Build history of the part. All positions in model axes, mm. A direction names the side the tool comes from. Give positions to 0.01 mm unless a question says otherwise; leave off trailing zeros. Order: outer loops, then holes, each group sorted by start corner. A loop starts at its lowest first (then second) coordinate and runs counter-clockwise, first axis right, second up. Notation, with made-up numbers: (34.5, -29.75) - (78.5, -29.75) arc R11 ccw to (78.5, -23.75) - close; hole circle Ø2 at (26, 79.5). An arc over 180 degrees is marked (long way). Use a Markdown table: item, result. Add a question column.
(1) Flat gauge pins, fed straight in: pin 1 (2 mm diameter, centred on y = 2.5, z = 2.5, fed in from -X); pin 2 (2 mm diameter, centred on y = -2, z = 3, fed in from -X); pin 3 (1.5 mm diameter, centred on y = 12.5, z = 2.5, fed in from -X). Where does each tip first touch, or does it go through?
(2) Which spindle directions (+Z, -Z, +X, -X, +Y, -Y) get a long thin tool onto all of the face, cutting with end or side? Do faces 5 (the face through (87.997, 12, 2)), 6 (the face through (53, -11, 2)). Say none if no direction does.
(3) Mould opens along Y. For faces 1 (the face through (60.003, -2, 2)), 2 (the face through (61.817, -21.617, 2.028)), 3 (the face through (42.246, 12.651, 1.972)), 4 (the face through (51.124, 26.516, 2.028)) say: +Y half, -Y half, draft (parallel to the pull), parting line (faces both ways), or undercut.
(4) Slice it at B-B (y = 11). Write the cut outline in (x, z), then the cut area to 3 significant figures.
(5) Wall check: line 1 (Y direction, x = 65.5, z = 0.6); line 2 (X direction, y = 1.5, z = 2.9); line 3 (X direction, y = 10.5, z = 0.35). Give the ranges that are in metal, low to high.
(6) Slice it at A-A (x = 40.5). Write the cut outline in (y, z), then the cut area to 3 significant figures.
(7) Slice it at D-D (y = -7). Write the cut outline in (x, z), then the cut area to 3 significant figures.
(8) Slice it at C-C (z = 1.85). Count the separate pieces of the cut face and the enclosed holes in it, then the cut area to 3 significant figures.
from build123d import *

# Parameters (mm, degrees)
SKETCH_3_R          = 2.1
EXTRUDE_2_DEPTH     = 4
FILLET_1_R          = 5
FILLET_3_R          = 6
FILLET_4_R          = 10
FILLET_5_R          = 35
CUT_EXTRUDE_START   = -4
SKETCH_4_R          = 1.6
SKETCH_4_R_2        = 2.1
CUT_EXTRUDE_1_DEPTH = 4
SKETCH_5_R          = 1.6
CUT_EXTRUDE_2_DEPTH = 4
FILLET_7_R          = 2
FILLET_8_R          = 2
FILLET_9_R          = 3
SKETCH_7_R          = 1.6
CUT_EXTRUDE_3_DEPTH = 10


with BuildPart() as part:
    # 草图3 → 凸台-拉伸2 (new body)
    with BuildSketch(Plane.XY):
        with BuildLine():
            Line((20.996765446, 45.242348331), (12.996765446, 35.70831959))
            ThreePointArc((12.996765446, 35.70831959), (31.127777683, 21.795904581), (38, 0))
            ThreePointArc((38, 0), (35.633322615, -13.20099691), (28.828088452, -24.757651669))
            Line((28.828088452, -24.757651669), (62.996765446, -24.757651669))
            Line((62.996765446, -24.757651669), (87.996765446, 3.242348331))
            Line((87.996765446, 3.242348331), (87.996765446, 23.242348331))
            Line((87.996765446, 23.242348331), (50.996765446, 26.242348331))
            Line((50.996765446, 26.242348331), (20.996765446, 45.242348331))
        make_face()
        with Locations((36.955694518, -19.956869561)):
            Circle(SKETCH_3_R, mode=Mode.SUBTRACT)
        with Locations((19.956869561, 36.955694518)):
            Circle(SKETCH_3_R, mode=Mode.SUBTRACT)
        with Locations((40.243259995, 12.019984399)):
            Circle(SKETCH_3_R, mode=Mode.SUBTRACT)
    extrude(amount=EXTRUDE_2_DEPTH)

    # 圆角1
    fillet_1_edges = [part.edges().sort_by_distance(p)[0] for p in [
        (20.996765446, 45.242348331, 2),
    ]]
    fillet(fillet_1_edges, radius=FILLET_1_R)

    # 圆角3
    fillet_3_edges = [part.edges().sort_by_distance(p)[0] for p in [
        (87.996765446, 23.242348331, 2),
        (87.996765446, 3.242348331, 2),
    ]]
    fillet(fillet_3_edges, radius=FILLET_3_R)

    # 圆角4
    fillet_4_edges = [part.edges().sort_by_distance(p)[0] for p in [
        (50.996765446, 26.242348331, 2),
    ]]
    fillet(fillet_4_edges, radius=FILLET_4_R)

    # 圆角5
    fillet_5_edges = [part.edges().sort_by_distance(p)[0] for p in [
        (62.996765446, -24.757651669, 2),
    ]]
    fillet(fillet_5_edges, radius=FILLET_5_R)

    # 草图4 → 切除-拉伸1 (cut)
    with BuildSketch(Plane.XY.offset(4).offset(CUT_EXTRUDE_START)):
        with Locations((55.003259995, 16.999984399)):
            Circle(SKETCH_4_R)
        with Locations((40.243259995, 12.019984399)):
            Circle(SKETCH_4_R_2)
        with Locations((85.003259995, 16.999984399)):
            Circle(SKETCH_4_R)
    extrude(amount=CUT_EXTRUDE_1_DEPTH, mode=Mode.SUBTRACT)

    # 草图5 → 切除-拉伸2 (cut)
    with BuildSketch(Plane.XY.offset(4).offset(CUT_EXTRUDE_START)):
        with Locations((55.003259995, 16.999984399)):
            Circle(SKETCH_5_R)
        Polygon((65.003259995, 11.999984399), (81.003259995, 11.999984399), (65.003259995, -10.000015601), align=None)
        Polygon((60.003259995, 10.999984399), (60.003259995, -11.000015601), (44.003259995, -11.000015601), align=None)
    extrude(amount=CUT_EXTRUDE_2_DEPTH, mode=Mode.SUBTRACT)

    # 圆角7
    fillet_7_edges = [part.edges().sort_by_distance(p)[0] for p in [
        (65.003259995, 11.999984399, 2),
        (60.003259995, -11.000015601, 2),
    ]]
    fillet(fillet_7_edges, radius=FILLET_7_R)

    # 圆角8
    fillet_8_edges = [part.edges().sort_by_distance(p)[0] for p in [
        (65.003259995, -10.000015601, 2),
        (81.003259995, 11.999984399, 2),
        (44.003259995, -11.000015601, 2),
        (60.003259995, 10.999984399, 2),
    ]]
    fillet(fillet_8_edges, radius=FILLET_8_R)

    # 圆角9
    fillet_9_edges = [part.edges().sort_by_distance(p)[0] for p in [
        (12.996765446, 35.70831959, 2),
        (28.828088452, -24.757651669, 2),
    ]]
    fillet(fillet_9_edges, radius=FILLET_9_R)

    # 草图7 → 切除-拉伸3 (cut)
    with BuildSketch(Plane.XY.offset(4)):
        with Locations((66.003259995, -11.000015601)):
            Circle(SKETCH_7_R)
    extrude(amount=-CUT_EXTRUDE_3_DEPTH, mode=Mode.SUBTRACT)


solid = part.part
Solution:
| question | item | result |
|---|---|---|
| 1 | pin 1 | x = 37.84 |
| 1 | pin 2 | x = 37.88 |
| 1 | pin 3 | x = 35.62 |
| 2 | face 5 | +Z, -Z, +X, +Y, -Y |
| 2 | face 6 | +Z, -Z |
| 3 | face 1 | undercut |
| 3 | face 2 | -Y half |
| 3 | face 3 | undercut |
| 3 | face 4 | +Y half |
| 4 | outline | (36.37, 0) - (38.41, 0) - (38.41, 4) - (36.37, 4) - close; (42.08, 0) - (65.27, 0) - (65.27, 4) - (42.08, 4) - close; (78.81, 0) - (88, 0) - (88, 4) - (78.81, 4) - close |
| 4 | area | 138 mm2 |
| 5 | line 1 | -19.67 to -12.52, -9.48 to -5.17, 11.32 to 25.07 |
| 5 | line 2 | 37.97 to 53.09, 60 to 65, 73.37 to 86.44 |
| 5 | line 3 | 36.52 to 38.79, 41.69 to 65.07, 79.01 to 88 |
| 6 | outline | (-24.76, 0) - (9.94, 0) - (9.94, 4) - (-24.76, 4) - close; (14.1, 0) - (32.89, 0) - (32.89, 4) - (14.1, 4) - close |
| 6 | area | 214 mm2 |
| 7 | outline | (37.35, 0) - (46.91, 0) - (46.91, 4) - (37.35, 4) - close; (60, 0) - (78.85, 0) - (78.85, 4) - (60, 4) - close |
| 7 | area | 114 mm2 |
| 8 | separate pieces | 1 |
| 8 | enclosed holes | 8 |
| 8 | area | 2,170 mm2 |
